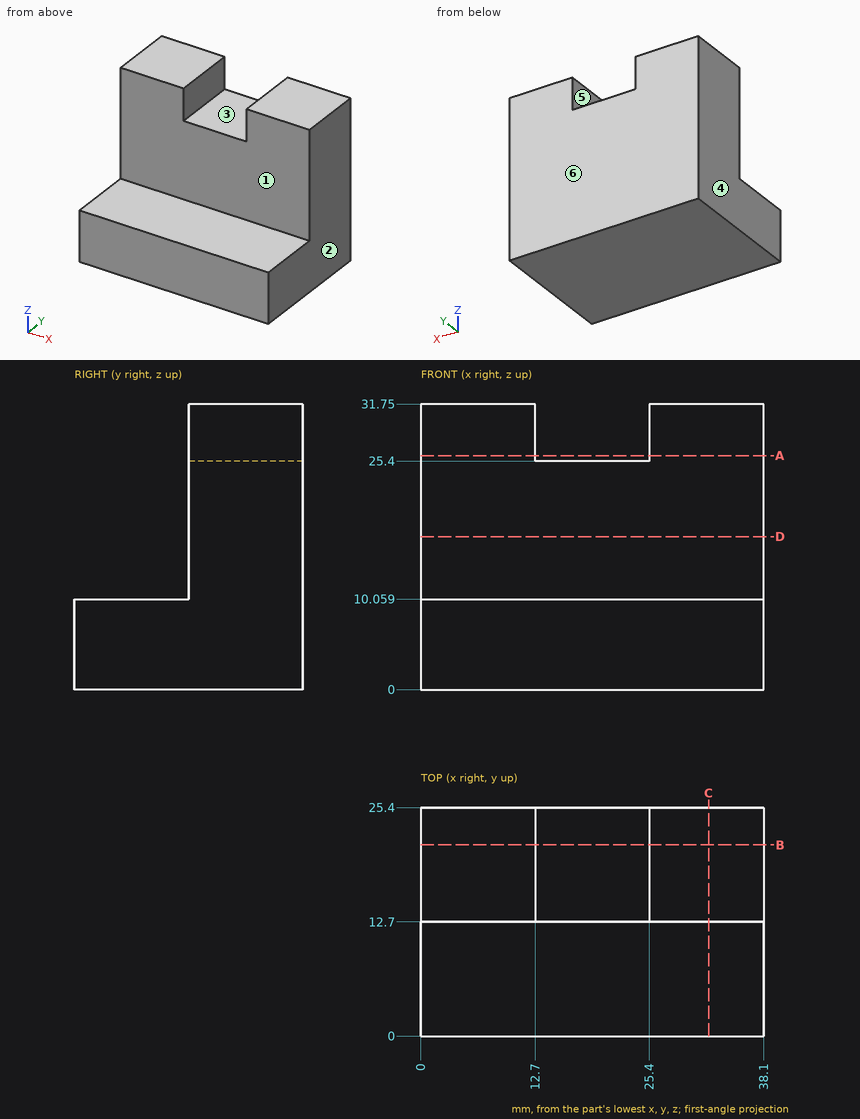
The drawing under review shows one solid part. Ordinate dimensions are in mm from its lowest x, y, z. A direction names the side the tool comes from. Give positions to 0.01 mm unless a question says otherwise; leave off trailing zeros. Loops run counter-clockwise (first coordinate to the right, second up) from the corner with the lowest first, then second, coordinate; pieces in that order, holes last. Notation, with made-up numbers: M -25,59 L -18,59 A30 cw -18,87 Z; hole C 78.25,81.5 d9. An arc over 180 degrees is marked long. Return JSON: item names as keys, results as strings. Group by question number.
Item 1: For probe 1 along Z at (x, y) = (14, 21.25); probe 2 along Z at (x, y) = (33.5, 7.25); probe 3 along X at (y, z) = (17.25, 29.5), list the stretches that pass through material, from the lowest coordinate up.
Item 2: Mouldability with a two-part tool opening along X and no side actions: class the marked faces 4, 5 and 6 as released by +X, released by -X, zero draft, split by the parting line, or undercut.
Item 3: Tool access review of the marked faces 1, 2 and 3: name each direction out of +Z, -Z, +X, -X, +Y, -Y from which nothing blocks a thin tool from reaching the whole face with its end or side.
Item 4: We need section D-D (z = 17). Give the boundary of the cut face in (x, y).
Item 5: We need section B-B (y = 21.25). Give the boundary of the cut face in (x, z), and give its area (3 significant figures).
Item 6: Insertion check: pin 1 Ø2 at (x, y) = (16, 13) entering from +Z; pin 2 Ø1.9 at (y, z) = (20.5, 29) entering from -X; pin 3 Ø14 at (x, y) = (16.5, 5.5) entering from +Z; pin 4 Ø4 at (x, z) = (29, 20) entering from -Y. Each pin has a flat end and moves straight along its axis. Give the tip position at first contact, or say it passes through.
Item 7: We need section C-C (x = 32). Give the boundary of the cut face in (y, z).
Item 8: We need section A-A (z = 26). Give the boundary of the cut face in (x, y).
Output:
{
 "1": {"probe 1": "z = 0 to 25.4", "probe 2": "z = 0 to 10.06", "probe 3": "x = 0 to 12.7, 25.4 to 38.1"},
 "2": {"face 4": "released by -X", "face 5": "undercut", "face 6": "zero draft"},
 "3": {"face 1": "+Z, +X, -X, -Y", "face 2": "+Z, -Z, +X, +Y, -Y", "face 3": "+Z, +Y, -Y"},
 "4": {"outline": "M 0,12.7 L 38.1,12.7 L 38.1,25.4 L 0,25.4 Z"},
 "5": {"outline": "M 0,0 L 38.1,0 L 38.1,31.75 L 25.4,31.75 L 25.4,25.4 L 12.7,25.4 L 12.7,31.75 L 0,31.75 Z", "area": "1,130 mm^2"},
 "6": {"pin 1": "stops at z = 25.4", "pin 2": "stops at x = 0", "pin 3": "stops at z = 10.06", "pin 4": "stops at y = 12.7"},
 "7": {"outline": "M 0,0 L 25.4,0 L 25.4,31.75 L 12.7,31.75 L 12.7,10.06 L 0,10.06 Z"},
 "8": {"outline": "M 0,12.7 L 12.7,12.7 L 12.7,25.4 L 0,25.4 Z; M 25.4,12.7 L 38.1,12.7 L 38.1,25.4 L 25.4,25.4 Z"}
}
